Study the drawing (mm; zero at the part's minimum x, y, z) and answer. Coordinates: 2 decimals unless noted, no trailing zeros. Order: outer loops, then holes, each group sorted by start corner. A loop starts at its lowest first (then second) coordinate and runs counter-clockwise, first axis right, second up. Notation, with made-up numbers: (19.25, 7.25) -> (52.25, 7.25) arc R5 cw to (52.25, 16.25) -> close; hole circle Ø7 at (36.5, -28.75). An arc over 180 degrees is marked (long way). Write each question's results on one line, items separated by ' | '. Start each with the question number.
(1) Straight lines are drawn through the part: L1, parallel to Z at x = 72.5, y = 0.7; L2, parallel to X at y = 1.25, z = 72.5; L3, parallel to X at y = 2.65, z = 52. For each, find the intervals that lie inside material, in ascending order.
(2) The part is cut by section A-A, the plane x = 7.5. Give the vertices of the cut face in (y, z).
(3) The part is cut by section B-B, the plane z = 72.5. Give the vertices of the cut face in (x, y).
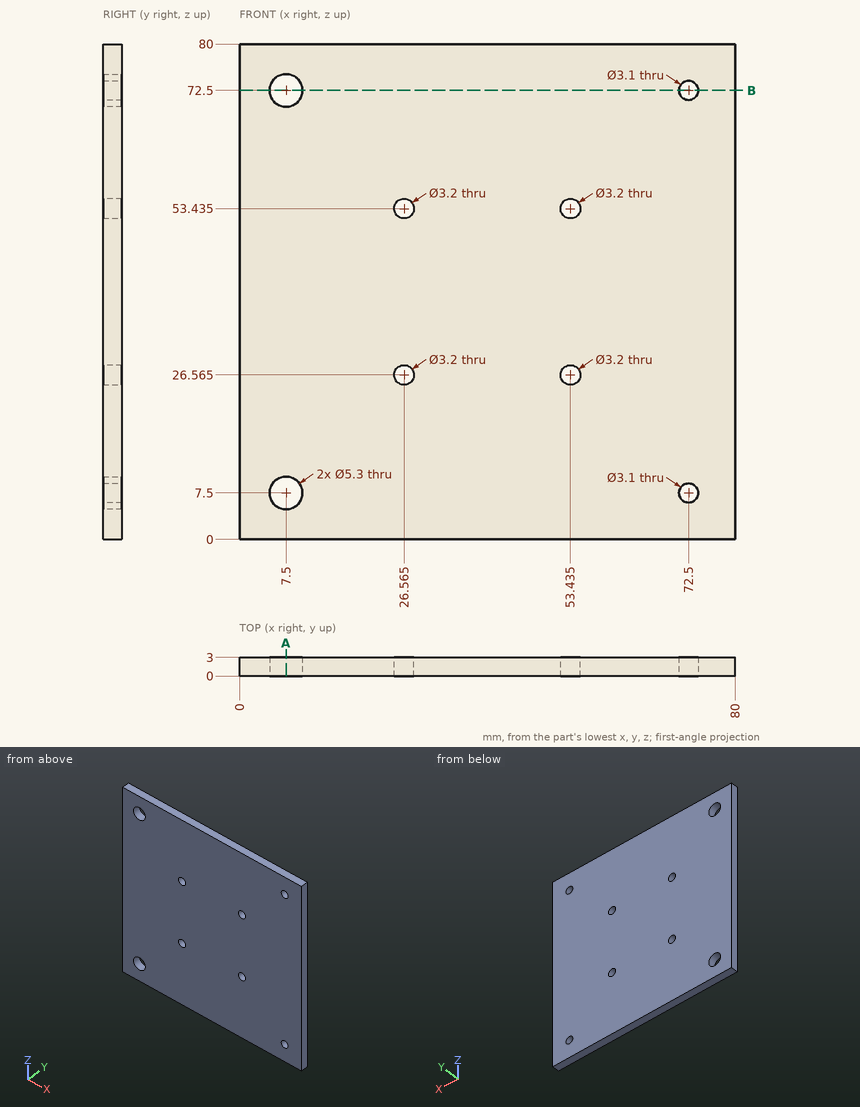
Established:
1) L1: z = 0 to 5.95, 9.05 to 70.95, 74.05 to 80 | L2: x = 0 to 4.85, 10.15 to 70.95, 74.05 to 80 | L3: x = 0 to 25.86, 27.27 to 52.73, 54.14 to 80
2) outline: (0, 0) -> (3, 0) -> (3, 4.85) -> (0, 4.85) -> close; (0, 10.15) -> (3, 10.15) -> (3, 69.85) -> (0, 69.85) -> close; (0, 75.15) -> (3, 75.15) -> (3, 80) -> (0, 80) -> close
3) outline: (0, 0) -> (4.85, 0) -> (4.85, 3) -> (0, 3) -> close; (10.15, 0) -> (70.95, 0) -> (70.95, 3) -> (10.15, 3) -> close; (74.05, 0) -> (80, 0) -> (80, 3) -> (74.05, 3) -> close
